from build123d import *

# Parameters (mm, degrees)
FILLET1_R   = 0.25
FILLET2_R   = 0.6
HEX_2_DEPTH = 3


with BuildPart() as part:
    # BodySke → Base-Revolve (revolve)
    with BuildSketch(Plane.XY, mode=Mode.PRIVATE) as base_revolve_sk:
        Polygon((0, 0), (0, 5), (4, 5), (4, 3), (13.4455, 3), (14, 2.4455), (14, 0), align=None)
    revolve(base_revolve_sk.sketch.rotate(Axis((-31.75, 0, 0), (1, 0, 0)), 90), axis=Axis((-31.75, 0, 0), (1, 0, 0)))  # turned: the seam where the file's is

    # Fillet1
    fillet1_edges = [part.edges().sort_by_distance(p)[0] for p in [
        (4, 0, -3),
    ]]
    fillet(fillet1_edges, radius=FILLET1_R)

    # Fillet2
    fillet2_edges = [part.edges().sort_by_distance(p)[0] for p in [
        (0, 0, -5),
    ]]
    fillet(fillet2_edges, radius=FILLET2_R)

    # Sketch2 → Hex-PreBroach (revolve, cut)
    with BuildSketch(Plane.XY, mode=Mode.PRIVATE) as hex_prebroach_sk:
        Polygon((0, 2), (3, 2), (4.154700538, 0), (0, 0), align=None)
    revolve(hex_prebroach_sk.sketch.rotate(Axis((0, 0, 0), (1, 0, 0)), 90), axis=Axis((0, 0, 0), (1, 0, 0)), mode=Mode.SUBTRACT)  # turned: the seam where the file's is

    # Sketch3 → Hex 2 (cut)
    with BuildSketch(Plane(origin=(0, 0, 0), x_dir=(0, 0.5, 0.866025404), z_dir=(-1, 0, 0))):
        Polygon((1.154700538, 2), (-1.154700538, 2), (-2.309401077, 0), (-1.154700538, -2), (1.154700538, -2), (2.309401077, 0), align=None)
    extrude(amount=-HEX_2_DEPTH, mode=Mode.SUBTRACT)


solid = part.part
Can you work these out from the model? Positions are in its coordinate system, mm. A direction names the side the tool comes from. Give positions to 0.01 mm unless a question says otherwise; leave off trailing zeros. Order: outer loops, then holes, each group sorted by start corner. A loop starts at its lowest first (then second) coordinate and runs counter-clockwise, first axis right, second up. Notation, with made-up numbers: M 3,85.5 L 23,85.5 A19 ccw 23,97.5 Z; hole C -15,80.5 d2. An arc over 180 degrees is marked long. One line per question, with ' | ' between items.
Item 1: For faces 1 (the face through (4, 1, 3.3)), 2 (the face through (2, 0, -5)), 3 (the face through (1.479, -1.724, -1.014)), which set-ups out of +Z, -Z, +X, -X, +Y, -Y let a thin tool reach every point of the face, with its end or its side?
Answer block:
face 1: +X | face 2: +X, -X | face 3: -X
Item 2: Please list where these lines run through material, in increasing order: L1, parallel to X at y = 3.75, z = 2; L2, parallel to Z at x = 4.25, y = -2; L3, parallel to Z at x = 1.75, y = -4.25.
Answer block:
L1: x = 0 to 4 | L2: z = -2.24 to 2.24 | L3: z = -2.63 to 2.63
Item 3: Suppose I cut it at A-A, the plane x = 9. Write out the boundary of the cut face in (y, z), then the cut area to 3 significant figures.
Answer block:
outline: C 0,0 d6 | area: 28.3 mm2
Item 4: We'd pull the mould along Y, two halves only. Please class faces 4 (the face through (8.91, -0.9, 2.86)), 5 (the face through (1.479, 1.724, 1.014)), 6 (the face through (14, 0, 0)): released by +Y, released by -Y, zero draft, split by the parting line, or undercut.
Answer block:
face 4: split by the parting line | face 5: undercut | face 6: zero draft
Item 5: I'm going to push flat-ended pins straight in: pin 1 Ø3 at (y, z) = (0, -2.5) entering from -X; pin 2 Ø4 at (x, z) = (10, -3) entering from -Y; pin 3 Ø1 at (y, z) = (-4, -3.5) entering from -X; pin 4 Ø6 at (x, z) = (10, -0.5) entering from -Y. Where does each tip first touch, or does it pass through?
Answer block:
pin 1: stops at x = 0 | pin 2: stops at y = -2.83 | pin 3: stops at x = 0.17 | pin 4: stops at y = -3
